Can you work these out from the model? Positions are in its coordinate system, mm. Face numbers are marked on the shaded views. A direction names the side the tool comes from. Give positions to 0.01 mm unless a question says otherwise; leave off trailing zeros. Order: outer loops, then holes, each group sorted by start corner. A loop starts at its lowest first (then second) coordinate and runs counter-clockwise, first axis right, second up. Notation, with made-up numbers: (35, -8) - (68, -8) arc R30 ccw to (68, 14) - close; hole circle Ø5 at (88.5, 2). An arc over 180 degrees is marked (long way). One line per question, with ' | ' between items.
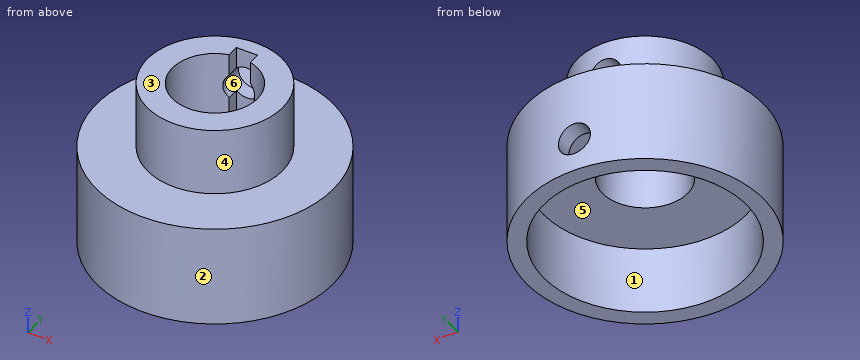
Autodesk Inventor part; units mm, degrees
ref_plane "YZ Plane" through (0, 0, 0) normal (1, 0, 0) x (0, 1, 0)
ref_plane "XZ Plane" through (0, 0, 0) normal (0, 1, 0) x (-1, 0, 0)
ref_plane "XY Plane" through (0, 0, 0) normal (0, 0, 1) x (1, 0, 0)
sketch "Sketch1" plane through (0, 0, 0) normal (0, 0, 1) x (1, 0, 0)
  circle A0 centre (0, 0) radius 9.525
  circle A1 centre (0, 0) radius 11.1125
  circle A2 centre (0, 0) radius 4
  circle A3 centre (0, 0) radius 6.35
  line L0 (-1, 3) -> (1, 3)
  line L1 (1, 3) -> (1, 5)
  line L2 (1, 5) -> (-1, 5)
  line L3 (-1, 5) -> (-1, 3)
  dimension "d0" = 19.05
  dimension "d1" = 22.225
  dimension "d2" = 8
  dimension "d3" = 12.7
  dimension "d15" = 2
  dimension "d16" = 2
  dimension "d17" = 1
  dimension "d18" = 5
extrude "Extrusion1" add sketch "Sketch1" along normal blind 3.175 contours A0 | A1 | A2 L3 L2 L1 | A3
extrude "Extrusion2" add sketch "Sketch1" along normal blind 9.525 contours A3
extrude "Extrusion3" add sketch "Sketch1" against normal blind 6.35 contours A1
sketch "Sketch2" plane through (0, 0, 0) normal (0, 1, 0) x (-1, 0, 0)
  circle A0 centre (0, 6.35) radius 1.5
  circle A1 centre (0, -3.175) radius 1.5
  line L0 (-9.525, 0) -> (9.525, 0)
  line L1 (-4, 9.525) -> (4, 9.525)
  point P0 (0, 0)
  point P1 (0, 0)
  dimension "d10" = 3
  dimension "d11" = 3.175
  dimension "d12" = 3.175
extrude "Extrusion4" cut sketch "Sketch2" along normal through all
equation "\"d16\" = d15"
properties part number "sprocket hub adaptor"
(1) If I drill on line 1 (Z direction, x = 0, y = 10.45) (3 decimals); line 2 (Z direction, x = 0, y = 5.5) (3 decimals); line 3 (X direction, y = -0.25, z = -2.25), over which ranges is the centre line in solid material (lowest first)?
Answer below:
line 1: -6.35 to -4.675, -1.675 to 3.175 | line 2: 0 to 4.85, 7.85 to 9.525 | line 3: -11.11 to -9.52, 9.52 to 11.11
(2) Imagine slicing it at A-A (x = 0). Count the separate pieces of the cut face and the enclosed holes in it, and give its area (3 significant figures).
Answer below:
separate pieces: 4 | enclosed holes: 0 | area: 80.0 mm^2
(3) Will these pins go through, and if not, where does the flat tip stop? pin 1 (0.9 mm diameter, centred on y = 4.5, z = 8.5, fed in from -X); pin 2 (6 mm diameter, centred on y = -5.5, z = -3, fed in from +X); pin 3 (2.5 mm diameter, centred on x = 0, z = 6.35, fed in from +Y).
Answer below:
pin 1: x = -4.89 | pin 2: x = 10.83 | pin 3: y = -3.8
(4) If we mould it in two halves opening along Y, with no side actions, what happens to the marked faces 1, 2 and 3? For each: released by +Y, released by -Y, zero draft, split by the parting line, or undercut.
Answer below:
face 1: undercut | face 2: split by the parting line | face 3: zero draft
(5) Imagine slicing it at C-C (y = 1.5). List the corners of the cut face in (x, z) for me (3 decimals).
Answer below:
outline: (-11.011, -6.35) - (-9.406, -6.35) - (-9.406, 0) - (-3.708, 0) - (-3.708, 9.525) - (-6.17, 9.525) - (-6.17, 3.175) - (-11.011, 3.175) - close; (3.708, 0) - (9.406, 0) - (9.406, -6.35) - (11.011, -6.35) - (11.011, 3.175) - (6.17, 3.175) - (6.17, 9.525) - (3.708, 9.525) - close
(6) Imagine slicing it at D-D (y = -7). List the corners of the cut face in (x, z) for me (3 decimals), and give its area (3 significant figures).
Answer below:
outline: (-8.631, -6.35) - (-6.46, -6.35) - (-6.46, 0) - (6.46, 0) - (6.46, -6.35) - (8.631, -6.35) - (8.631, 3.175) - (-8.631, 3.175) - close | area: 82.4 mm^2
(7) On a 3-axis mill with a long thin cutter (end or side, diameter ignored), from which of +Z, -Z, +X, -X, +Y, -Y can I reach the whole of each face in a straight line? I mean the marked faces 4, 5 and 6. Say none if no direction works.
Answer below:
face 4: +Z | face 5: -Z | face 6: +Y
